The listing builds one solid part. Answer for the finished solid, in the listing's coordinates (mm). Round coordinates to 2 decimals unless told otherwise and drop trailing zeros. Order: outer loops, then holes, each group sorted by start corner. A loop starts at its lowest first (then second) coordinate and runs counter-clockwise, first axis right, second up. Notation, with made-up numbers: (-31.75, 84) -> (18.25, 84) arc R3 ccw to (18.25, 88) -> close; hole circle Ø9 at (-34.5, 70.25). An arc over 180 degrees is marked (long way). Answer in a Markdown table with one row per item. Add a question column.
Autodesk Inventor part; units mm, degrees
ref_plane "YZ Plane" through (0, 0, 0) normal (1, 0, 0) x (0, 1, 0)
ref_plane "XZ Plane" through (0, 0, 0) normal (0, 1, 0) x (-1, 0, 0)
ref_plane "XY Plane" through (0, 0, 0) normal (0, 0, 1) x (1, 0, 0)
sketch "Esquisse1" plane through (0, 0, 0) normal (0, 1, 0) x (-1, 0, 0)
  line L0 (23.7435, 85.6153) -> (3.7435, 85.6153)
  line L1 (3.7435, 85.6153) -> (3.7435, -14.3847)
  line L2 (3.7435, -14.3847) -> (23.7435, -14.3847)
  line L3 (23.7435, -14.3847) -> (23.7435, 85.6153)
  point P0 (0, 0)
  dimension "d0" = 100
  dimension "d1" = 20
extrude "Extrusion1" add sketch "Esquisse1" along normal blind 5
sketch "Esquisse2" plane through (0, 5, 0) normal (0, 1, 0) x (1, 0, 0)
  circle A0 centre (-13.7435, 3.3847) radius 4
  line L0 (-3.7435, 14.3847) -> (-23.7435, 14.3847)
  line L1 (-3.7435, -85.6153) -> (-3.7435, 14.3847)
  circle A1 centre (-13.7435, 11.3847) radius 1.5
  circle A2 centre (-5.7435, 3.3847) radius 1.5
  circle A3 centre (-21.7435, 3.3847) radius 1.5
  line L2 (-23.7435, 14.3847) -> (-23.7435, -85.6153)
  circle A4 centre (-13.7435, -4.6153) radius 1.5
  point P0 (0, 0)
  dimension "d4" = 11
  dimension "d5" = 10
  dimension "d6" = 8
  dimension "d9" = 3
  dimension "d10" = 3
  dimension "d11" = 10
  dimension "d12" = 2
  dimension "d13" = 3
  dimension "d14" = 11
  dimension "d15" = 2
  dimension "d16" = 11
  dimension "d17" = 3
  dimension "d18" = 10
  dimension "d19" = 3
  dimension "d20" = 19
extrude "Extrusion2" cut sketch "Esquisse2" against normal through all
properties part number "bras-lanceur"
Item 1: The part is cut by section B-B, the plane y = 2.95. Give the vertices of the cut face in (x, z), and give its area (3 significant figures).
Item 2: The part is cut by section C-C, the plane x = -13.25. Give the vertices of the cut face in (y, z), and give its area (3 significant figures).
Item 3: For a pull along X with two mould halves and no side action, classify faces 1 (the face through (-23.744, 2, 35)), 2 (the face through (-14, 2, -14.385)), 3 (the face through (-12.313, 2.535, 4.165)), 4 (the face through (-3.744, 2, 36)) as released by +X, released by -X, zero draft, split by the parting line, or undercut.
Item 4: Flat-ended cylindrical pins translate along their axes: P1, Ø5, axis at x = -13.74, z = -11.38, coming from the +Y side; P2, Ø2.5, axis at x = -13.74, z = 4.62, coming from the -Y side. Find the tip coordinate at first contact, or state that the pin passes through.
Item 5: The part is cut by section A-A, the plane x = -22. Give the vertices of the cut face in (y, z), and give its area (3 significant figures).
Item 6: Find the intervals of material crossed by probe 1 along Z at (x, y) = (-21.5, 3.45); probe 2 along X at (y, z) = (4.5, -7); probe 3 along Z at (x, y) = (-16.5, 2), in increasing order. Write a range as [from, to].
Resolved:
| question | item | result |
|---|---|---|
| 1 | outline | (-23.74, -14.38) -> (-3.74, -14.38) -> (-3.74, 85.62) -> (-23.74, 85.62) -> close; hole circle Ø3 at (-21.74, -3.38); hole circle Ø8 at (-13.74, -3.38); hole circle Ø3 at (-13.74, -11.38); hole circle Ø3 at (-13.74, 4.62); hole circle Ø3 at (-5.74, -3.38) |
| 1 | area | 1,920 mm2 |
| 2 | outline | (0, -14.38) -> (5, -14.38) -> (5, -12.8) -> (0, -12.8) -> close; (0, -9.97) -> (5, -9.97) -> (5, -7.35) -> (0, -7.35) -> close; (0, 0.58) -> (5, 0.58) -> (5, 3.2) -> (0, 3.2) -> close; (0, 6.03) -> (5, 6.03) -> (5, 85.62) -> (0, 85.62) -> close |
| 2 | area | 432 mm2 |
| 3 | face 1 | released by -X |
| 3 | face 2 | zero draft |
| 3 | face 3 | undercut |
| 3 | face 4 | released by +X |
| 4 | P1 | y = 5 |
| 4 | P2 | through |
| 5 | outline | (0, -14.38) -> (5, -14.38) -> (5, -4.86) -> (0, -4.86) -> close; (0, -1.91) -> (5, -1.91) -> (5, 85.62) -> (0, 85.62) -> close |
| 5 | area | 485 mm2 |
| 6 | probe 1 | [-14.38, -4.86], [-1.9, 85.62] |
| 6 | probe 2 | [-23.74, -15.46], [-12.03, -3.74] |
| 6 | probe 3 | [-14.38, -6.28], [-0.49, 85.62] |
